Autodesk Inventor part; units mm, degrees
ref_plane "YZ Plane" through (0, 0, 0) normal (1, 0, 0) x (0, 1, 0)
ref_plane "XZ Plane" through (0, 0, 0) normal (0, 1, 0) x (-1, 0, 0)
ref_plane "XY Plane" through (0, 0, 0) normal (0, 0, 1) x (1, 0, 0)
sketch "Sketch1" plane through (0, 0, 0) normal (1, 0, 0) x (0, 1, 0)
  line L0 (-232.9787, 228.8989) -> (-240.0787, 228.8989)
  line L1 (-240.0787, 228.8989) -> (-240.0787, 226.3489)
  line L2 (-240.0787, 226.3489) -> (-247.0787, 226.3489)
  line L3 (-261.0787, 231.3489) -> (-248.0787, 231.3489)
  line L4 (-232.9787, 228.8989) -> (-232.9787, 227.8989)
  line L5 (-232.9787, 227.8989) -> (-239.0787, 227.8989)
  line L6 (-239.0787, 227.8989) -> (-239.0787, 227.8489)
  line L7 (-258.789, 225.8489) -> (279.9992, 225.8489) construction
  line L8 (-232.9787, 222.7989) -> (-240.0787, 222.7989)
  line L9 (-240.0787, 222.7989) -> (-240.0787, 225.3489)
  line L10 (-240.0787, 225.3489) -> (-247.0787, 225.3489)
  line L11 (-261.0787, 220.3489) -> (-248.0787, 220.3489)
  line L12 (-232.9787, 222.7989) -> (-232.9787, 223.7989)
  line L13 (-232.9787, 223.7989) -> (-239.0787, 223.7989)
  line L14 (-239.0787, 223.7989) -> (-239.0787, 227.8489)
  line L15 (-248.0787, 231.3489) -> (-248.0787, 220.3489)
  line L16 (-261.0787, 231.3489) -> (-261.0787, 232.3489)
  line L17 (-261.0787, 232.3489) -> (-247.0787, 232.3489)
  line L18 (-247.0787, 232.3489) -> (-247.0787, 226.3489)
  line L19 (-247.0787, 225.3489) -> (-247.0787, 219.3489)
  line L20 (-247.0787, 219.3489) -> (-261.0787, 219.3489)
  line L21 (-261.0787, 219.3489) -> (-261.0787, 220.3489)
  point P0 (0, 0)
  dimension "d4" = 1
  dimension "d6" = 4.1
  dimension "d9" = 1
  dimension "d10" = 1
  dimension "d13" = 6.1
  dimension "d14" = 11
  dimension "d15" = 1
  dimension "d16" = 1
  dimension "d17" = 1
  dimension "d29" = 13
  dimension "d32" = 7
extrude "Extrusion1" add sketch "Sketch1" along normal blind 8
sketch "Sketch2" plane through (0, -261.0787, 219.3489) normal (0, 0, -1) x (-1, 0, 0)
  line L0 (0, 14) -> (-8, 14)
  line L1 (0, 0) -> (0, 14)
  point P0 (0, 261.0787)
  point P1 (-4, 3)
  dimension "d25" = 11
  dimension "d26" = 4
  dimension "d27" = 8
  dimension "d28" = 14
hole "Hole1" at (4, -258.0787, 219.3489) direction (0, 0, 1) diameter 1.7 end through all
fillet "Fillet1" radius 0.5 4 edges at (4, -261.0787, 231.3489) (4, -261.0787, 232.3489) (4, -261.0787, 220.3489) (4, -261.0787, 219.3489)
fillet "Fillet2" radius 1 10 edges at (4, -247.0787, 232.3489) (4, -248.0787, 231.3489) (4, -247.0787, 219.3489) (4, -248.0787, 220.3489) (4, -247.0787, 225.3489) (4, -247.0787, 226.3489) (4, -240.0787, 226.3489) (4, -240.0787, 222.7989) (4, -240.0787, 225.3489) (4, -240.0787, 228.8989)
properties part number "back_wheel_interface"
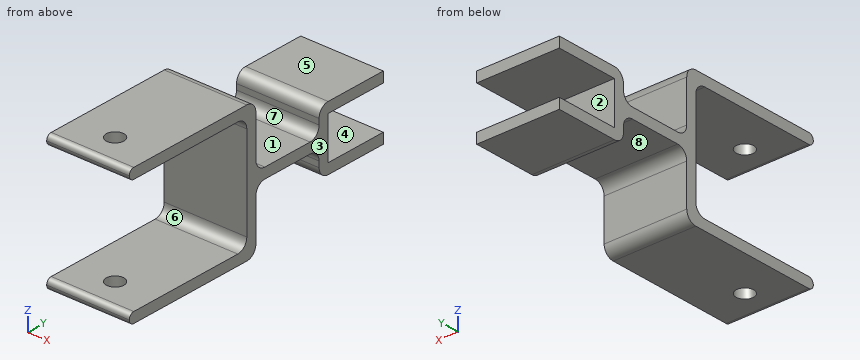
Work out the finished part from the listing and answer in its coordinate system (mm). Face numbers are marked on the shaded views. A direction names the side the tool comes from. Give positions to 0.01 mm unless a question says otherwise; leave off trailing zeros. Loops run counter-clockwise (first coordinate to the right, second up) from the corner with the lowest first, then second, coordinate; pieces in that order, holes last. Notation, with made-up numbers: (83, 62) -> (124, 62) arc R17 cw to (124, 78) -> close; hole circle Ø7 at (22.5, 74). An arc over 180 degrees is marked (long way). Use a Markdown table: item, result. Add a question column.
1) Each of these flat-tipped pins is pushed along its axis until it touches: P1, Ø3, axis at x = 5.5, z = 222.5, coming from the +Y side; P2, Ø1, axis at x = 1.5, z = 226.5, coming from the -Y side; P3, Ø1.8, axis at x = 5.5, y = -234.5, coming from the +Z side; P4, Ø4, axis at x = 6, y = -242.5, coming from the +Z side. Where does it stop, or does it pass through?
2) The part is cut by section D-D, the plane x = 4. Count the separate pieces of the cut face and the enclosed holes in it, plus the area to 3 significant figures.
3) The part is cut by section B-B, the plane z = 223.5. Determine the outline of the cut face in (x, y).
4) Which of the six approach directions +Z, -Z, +X, -X, +Y, -Y give full straight-line access (tool end or side, diameter ignored) to the marked faces 4, 5, 6, 7 and 8?
5) Consider line 1 along Z through (x, y) = (5, -256.5); line 2 along Z through (x, y) = (6.25, -238.75); line 3 along Z through (x, y) = (7.75, -244.25). Determine where each line is inside the solid, lowest interval first.
6) The part is cut by section A-A, the plane y = -251.25. Determine the outline of the cut face in (x, z).
7) For a pull along Z with two mould halves and no side action, classify the marked faces 1, 2 and 3 as +Z half, -Z half, draft (parallel to the pull), parting line (faces both ways), or undercut.
Reported:
| question | item | result |
|---|---|---|
| 1 | P1 | stops at y = -232.98 |
| 1 | P2 | stops at y = -248.08 |
| 1 | P3 | stops at z = 228.9 |
| 1 | P4 | stops at z = 226.53 |
| 2 | separate pieces | 3 |
| 2 | enclosed holes | 0 |
| 2 | area | 61.1 mm^2 |
| 3 | outline | (0, -248.08) -> (8, -248.08) -> (8, -247.08) -> (0, -247.08) -> close; (0, -240.03) -> (8, -240.03) -> (8, -232.98) -> (0, -232.98) -> close |
| 4 | face 4 | +X, -X, +Y |
| 4 | face 5 | +Z, +X, -X, +Y |
| 4 | face 6 | +X, -X, -Y |
| 4 | face 7 | +Z, +X, -X |
| 4 | face 8 | -Z, +X, -X |
| 5 | line 1 | z = 219.35 to 220.35, 231.35 to 232.35 |
| 5 | line 2 | z = 222.8 to 223.8, 227.9 to 228.9 |
| 5 | line 3 | z = 225.35 to 226.35 |
| 6 | outline | (0, 219.35) -> (8, 219.35) -> (8, 220.35) -> (0, 220.35) -> close; (0, 231.35) -> (8, 231.35) -> (8, 232.35) -> (0, 232.35) -> close |
| 7 | face 1 | +Z half |
| 7 | face 2 | undercut |
| 7 | face 3 | draft |
